Design review of the part shown in the three views and the two pictorial views. Dimensions are in mm from the part's minimum x, y and z. A direction names the side the tool comes from. Coordinates: 2 decimals unless noted, no trailing zeros. Order: outer loops, then holes, each group sorted by start corner. A loop starts at its lowest first (then second) coordinate and runs counter-clockwise, first axis right, second up. Notation, with made-up numbers: (-16.75, -21.75) -> (15.25, -21.75) arc R28 ccw to (15.25, 9.25) -> close; hole circle Ø9 at (-39.75, 47.25). An arc over 180 degrees is marked (long way). Answer as a JSON object with one key per item and string values. Group by question number.
1) Draft analysis for pull direction X (two halves, no side actions). For the marked faces 1, 2 and 3, state which applies: +X half, -X half, draft (parallel to the pull), parting line (faces both ways), or undercut.
2) Add section B-B, the plane x = 6. Write out the cut boundary in (y, z), then the cut area to 3 significant figures.
3) Add section D-D, the plane x = 8.5. Write out the cut boundary in (y, z), then the cut area to 3 significant figures.
4) Add section C-C, the plane y = 6.25. Write out the cut boundary in (x, z), then the cut area to 3 significant figures.
5) Add section A-A, the plane z = 3.5. Write out the cut boundary in (x, y), then the cut area to 3 significant figures.
6) For pin 1 (1 mm diameter, centred on x = 9.5, y = 6, fed in from -Z); pin 2 (1.5 mm diameter, centred on x = 6.5, z = 1.5, fed in from +Y); pin 3 (4 mm diameter, centred on x = 3.5, z = 5.5, fed in from +Y), all flat-tipped, find the tip position at first contact; note any pin that passes through.
7) Wall thickness on L1, parallel to Z at x = 5, y = 2.5; L2, parallel to Z at x = 9, y = 2.5; L3, parallel to Y at x = 6, z = 1: over which ranges is each line inside the solid? List them lowest first.
8) Machinability: for the marked faces 4, 5 and 6, which of the approach directions +Z, -Z, +X, -X, +Y, -Y give a long, thin tool a straight path to every point of the face, cutting with its end or side? Answer none if there is none.
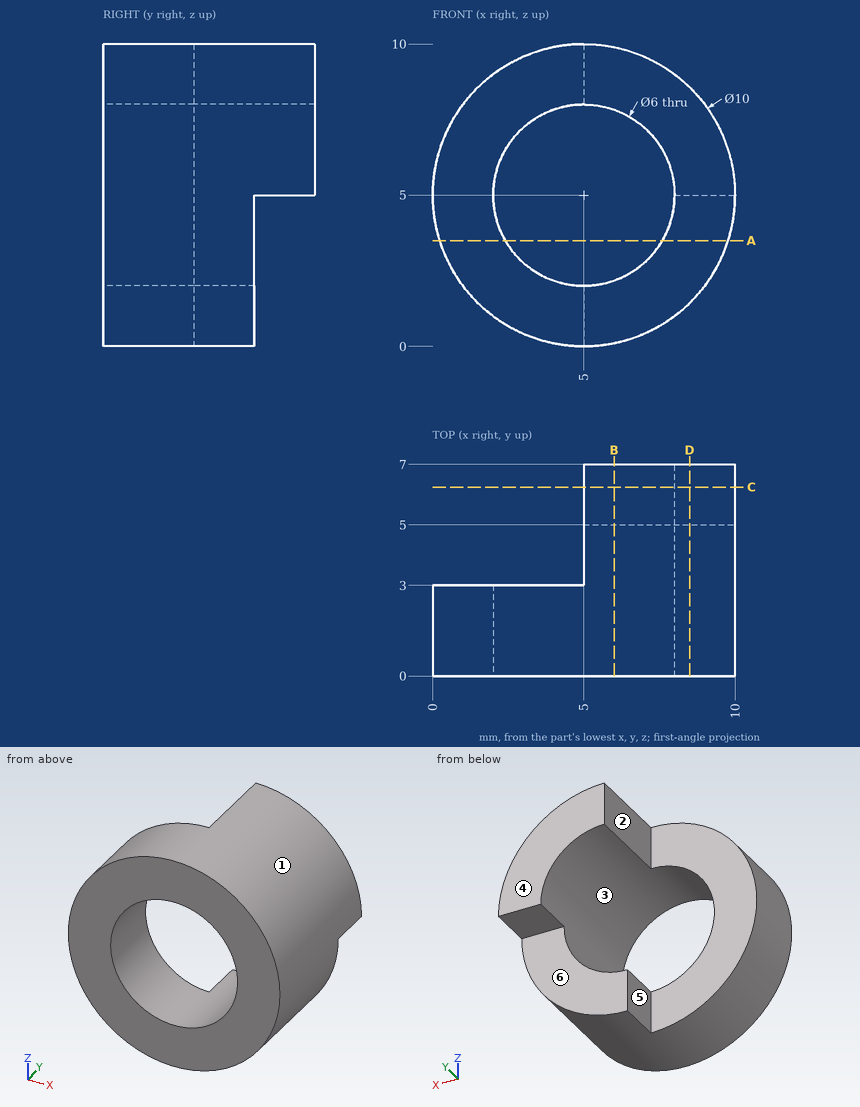
Output values:
{
 "1": {"face 1": "parting line", "face 2": "-X half", "face 3": "undercut"},
 "2": {"outline": "(0, 0.1) -> (5, 0.1) -> (5, 2.17) -> (0, 2.17) -> close; (0, 7.83) -> (7, 7.83) -> (7, 9.9) -> (0, 9.9) -> close", "area": "24.8 mm²"},
 "3": {"outline": "(0, 1.43) -> (5, 1.43) -> (5, 5) -> (7, 5) -> (7, 8.57) -> (0, 8.57) -> close", "area": "42.8 mm²"},
 "4": {"outline": "(5, 8) arc R3 cw to (8, 5) -> (10, 5) arc R5 ccw to (5, 10) -> close", "area": "12.6 mm²"},
 "5": {"outline": "(0.23, 0) -> (2.4, 0) -> (2.4, 3) -> (0.23, 3) -> close; (7.6, 0) -> (9.77, 0) -> (9.77, 5) -> (7.6, 5) -> close", "area": "17.4 mm²"},
 "6": {"pin 1": "stops at z = 5", "pin 2": "stops at y = 5", "pin 3": "stops at y = 3"},
 "7": {"L1": "z = 0 to 2, 8 to 10", "L2": "z = 2 to 8", "L3": "y = 0 to 5"},
 "8": {"face 4": "+Z, -Z, +X, -X, +Y", "face 5": "+Z, -Z, -X, +Y", "face 6": "-Z, +X, -X, +Y"}
}
